The listing builds one solid part. Answer for the finished solid, in the listing's coordinates (mm). A direction names the side the tool comes from. Round coordinates to 2 decimals unless told otherwise and drop trailing zeros. Loops run counter-clockwise (first coordinate to the right, second up) from the corner with the lowest first, then second, coordinate; pieces in that order, holes last. Notation, with made-up numbers: (70.25, 26) - (110.25, 26) arc R34 cw to (110.25, 62) - close; hole circle Ø8 at (-38, 80.25). An arc over 180 degrees is marked (long way). Write item = value, one per line. Start each with the question number.
1) Section B-B, the plane z = -12 is taken. Determine the outline of the cut face in (x, y), and give its area (3 significant figures).
2) Section A-A, the plane z = 16.5 is taken. Determine the outline of the cut face in (x, y).
3) Section C-C, the plane y = 1.6 is taken. Give the number of separate pieces and of enclosed holes in the cut face, and give its area (3 significant figures).
4) A tool of negligible diameter and unlimited length cuts with its end or side. For faces 1 (the cylindrical face through (46.35, 1.52, -34.14)), 2 (the flat face through (-36, 2, 27)), 3 (the flat face through (25.75, 2, -18)), 4 (the flat face through (-37, 2, 31)), from which of +Z, -Z, +X, -X, +Y, -Y can it reach the whole face along a straight path? Write none if from no direction.
5) For a pull along X with two mould halves and no side action, classify faces 5 (the flat face through (-42, 1, 35)), 6 (the flat face through (-35.25, 2, 29)), 7 (the flat face through (47.25, 1, 30)) as released by +X, released by -X, zero draft, split by the parting line, or undercut.
6) Straight lines are drawn through the part: line 1 along X through (y, z) = (2.15, 31.5); line 2 along Z through (x, y) = (41, 0.95); line 3 along X through (y, z) = (0.9, -31.5). For each, find the intervals that lie inside material, in ascending order.
7) Given pin 1 Ø1.8 at (x, z) = (43.75, 31.5) entering from +Y; pin 2 Ø1 at (x, y) = (17.5, 2.5) entering from +Z, each flat-ended and moving along its own axis, determine where each tip first touches the part or whether it passes through.
8) Section D-D, the plane x = 5 is taken. Determine the outline of the cut face in (y, z).
from build123d import *

# Parameters (mm, degrees)
SKETCH1_W           = 94.5
SKETCH1_H           = 70
BOSS_EXTRUDE1_DEPTH = 3
SKETCH3_R           = 1.5
CUT_EXTRUDE2_DEPTH  = 59.877521177
FILLET2_R           = 3
SKETCH5_W           = 64
SKETCH5_H           = 56
SKETCH5_W_2         = 21.5
SKETCH5_H_2         = 18
SKETCH5_W_3         = 17.5
SKETCH5_H_3         = 15
CUT_EXTRUDE3_DEPTH  = 59.877521177
FILLET3_R           = 3


with BuildPart() as part:
    # Sketch1 → Boss-Extrude1 (new body)
    with BuildSketch(Plane(origin=(0, 0, 0), x_dir=(1, 0, 0), z_dir=(0, 1, 0))):
        Rectangle(SKETCH1_W, SKETCH1_H)
    extrude(amount=BOSS_EXTRUDE1_DEPTH)

    # Sketch3 → Cut-Extrude2 (cut, through all)
    with BuildSketch(Plane(origin=(0, 3, 0), x_dir=(1, 0, 0), z_dir=(0, 1, 0))):
        with Locations(Location((43.75, 31.5, 0), (0, 0, 270))):
            Circle(SKETCH3_R)
        with Locations(Location((-43.25, 31.5, 0), (0, 0, 270))):
            Circle(SKETCH3_R)
        with Locations(Location((-43.25, -31.5, 0), (0, 0, 270))):
            Circle(SKETCH3_R)
        with Locations(Location((43.75, -31.5, 0), (0, 0, 270))):
            Circle(SKETCH3_R)
    extrude(amount=-CUT_EXTRUDE2_DEPTH, mode=Mode.SUBTRACT)

    # Fillet2
    fillet2_edges = [part.edges().sort_by_distance(p)[0] for p in [
        (47.25, 1.5, 35),
        (-47.25, 1.5, 35),
        (-47.25, 1.5, -35),
        (47.25, 1.5, -35),
    ]]
    fillet(fillet2_edges, radius=FILLET2_R)

    # Sketch5 → Cut-Extrude3 (cut, through all)
    with BuildSketch(Plane(origin=(0, 3, 0), x_dir=(1, 0, 0), z_dir=(0, 1, 0))):
        with Locations((-8.25, 1)):
            Rectangle(SKETCH5_W, SKETCH5_H)
        with Locations((36.5, 18)):
            Rectangle(SKETCH5_W_2, SKETCH5_H_2)
        with Locations((38.5, -1.5)):
            Rectangle(SKETCH5_W_3, SKETCH5_H_3)
        with Locations((38.5, -19.5)):
            Rectangle(SKETCH5_W_3, SKETCH5_H_3)
        Polygon((17.75, -27), (-35.25, -27), (-35.25, -31), (-39.25, -31), (-39.25, -35), (20.75, -35), (20.75, -31), (17.75, -31), align=None)
    extrude(amount=-CUT_EXTRUDE3_DEPTH, mode=Mode.SUBTRACT)

    # Fillet3
    fillet3_edges = [part.edges().sort_by_distance(p)[0] for p in [
        (-40.25, 1.5, 27),
        (-40.25, 1.5, -29),
        (23.75, 1.5, -29),
        (23.75, 1.5, 27),
    ]]
    fillet(fillet3_edges, radius=FILLET3_R)


solid = part.part
Geometry check:
q1.outline = (-47.25, 0) - (-40.25, 0) - (-40.25, 3) - (-47.25, 3) - close; (23.75, 0) - (25.75, 0) - (25.75, 3) - (23.75, 3) - close
q1.area = 27.0 mm2
q2.outline = (-47.25, 0) - (-40.25, 0) - (-40.25, 3) - (-47.25, 3) - close; (23.75, 0) - (29.75, 0) - (29.75, 3) - (23.75, 3) - close
q3.separate_pieces = 1
q3.enclosed_holes = 4
q3.area = 1,640 mm2
q4.face_1 = -Z, +X, +Y, -Y
q4.face_2 = +Y, -Y
q4.face_3 = +X, +Y, -Y
q4.face_4 = +Z, +Y, -Y
q5.face_5 = zero draft
q5.face_6 = undercut
q5.face_7 = released by +X
q6.line_1 = -47.25 to -44.75, -41.75 to -39.25, 20.75 to 42.25, 45.25 to 47.25
q6.line_2 = -35 to -27, -9 to -6, 9 to 12, 27 to 35
q6.line_3 = -47.25 to -44.75, -41.75 to 42.25, 45.25 to 47.25
q7.pin_1 = through
q7.pin_2 = 31
q8.outline = (0, -35) - (3, -35) - (3, -29) - (0, -29) - close
